from build123d import *

# Parameters (mm, degrees)
SKETCH1_R           = 10
SKETCH1_R_2         = 7.5
BOSS_EXTRUDE1_DEPTH = 25
THREAD1_PITCH       = 0.3175
SKETCH4_W           = 146
SKETCH4_H           = 146
BOSS_EXTRUDE2_DEPTH = 2
SKETCH5_W           = 148
SKETCH5_H           = 148
BOSS_EXTRUDE3_DEPTH = 1
SKETCH6_W           = 10
SKETCH6_H           = 3
SKETCH6_R           = 1
BOSS_EXTRUDE4_DEPTH = 5
CHAMFER2_START      = -5
CHAMFER2_DEPTH      = 10
SKETCH9_R           = 10
CUT_EXTRUDE1_DEPTH  = 111.385687501
FILLET1_R           = 1


with BuildPart() as part:
    # Sketch1 → Boss-Extrude1 (new body)
    with BuildSketch(Plane(origin=(0, 0, 0), x_dir=(1, 0, 0), z_dir=(0, 1, 0))):
        with Locations(Location((0, 0, 0), (0, 0, 270))):
            Circle(SKETCH1_R)
        with Locations(Location((0, 0, 0), (0, 0, 270))):
            Circle(SKETCH1_R_2, mode=Mode.SUBTRACT)
    extrude(amount=BOSS_EXTRUDE1_DEPTH)

    # Thread1: arcs per turn and ends read off the stored shape
    # Thread1: the profile of Thread Profile1 profile screwed along a right-hand helix through 18.897638 turns, 6 arcs to a turn; built about Z, then put on its axis
    thread1_z = Axis((0, 0, 0), (0, 0, 1))
    thread1_corners = [(10.0003, 0, -0.000173205), (10.0003, 0, 0.277985704), (9.828148085, 0, 0.17859375), (9.828148085, 0, 0.09921875)]
    with BuildLine(mode=Mode.PRIVATE) as thread1_profile:
        Line(thread1_corners[0], thread1_corners[1])
        Line(thread1_corners[1], thread1_corners[2])
        Line(thread1_corners[2], thread1_corners[3])
        Line(thread1_corners[3], thread1_corners[0])
    thread1_cap = Face(thread1_profile.wire())
    thread1_turn_angles = [0, 30, 60, 90, 120, 150, 180, 210, 240, 270, 300, 330, 360]
    thread1_turn_weights = [1, 0.8660254037844387, 1, 0.8660254037844387, 1, 0.8660254037844387, 1, 0.8660254037844387, 1, 0.8660254037844387, 1, 0.8660254037844387, 1]
    thread1_turn_rails = [Edge.make_bspline([Vector(p[0], p[1], 0).rotate(thread1_z, thread1_turn_angles[k]) / thread1_turn_weights[k] + Vector(0, 0, p[2] + THREAD1_PITCH * thread1_turn_angles[k] / 360) for k in range(13)], [0, 0, 0, 1, 1, 2, 2, 3, 3, 4, 4, 5, 5, 6, 6, 6], 2, thread1_turn_weights) for p in thread1_corners]
    thread1_turn_sides = [Face.make_surface_from_curves(thread1_turn_rails[p[0]], thread1_turn_rails[p[1]]) for p in [(0, 1), (1, 2), (2, 3), (3, 0)]]
    thread1_last_angles = [6480, 6510, 6540, 6570, 6600, 6630, 6660, 6690, 6720, 6750, 6780, 6791.57480315, 6803.149606299]
    thread1_last_weights = [1, 0.8660254037844387, 1, 0.8660254037844387, 1, 0.8660254037844387, 1, 0.8660254037844387, 1, 0.8660254037844387, 1, 0.9796635825089068, 1]
    thread1_last_rails = [Edge.make_bspline([Vector(p[0], p[1], 0).rotate(thread1_z, thread1_last_angles[k]) / thread1_last_weights[k] + Vector(0, 0, p[2] + THREAD1_PITCH * thread1_last_angles[k] / 360) for k in range(13)], [0, 0, 0, 1, 1, 2, 2, 3, 3, 4, 4, 5, 5, 6, 6, 6], 2, thread1_last_weights) for p in thread1_corners]
    thread1_last_sides = [Face.make_surface_from_curves(thread1_last_rails[p[0]], thread1_last_rails[p[1]]) for p in [(0, 1), (1, 2), (2, 3), (3, 0)]]
    thread1 = Plane(origin=(0, -0.5, 0), x_dir=(1, 0, 0), z_dir=(0, 1, 0)) * Solid(Shell([*[p.moved(Location((0, 0, THREAD1_PITCH * i))) for i in range(18) for p in thread1_turn_sides], *thread1_last_sides, thread1_cap, thread1_cap.rotate(thread1_z, 6803.149606299).moved(Location((0, 0, THREAD1_PITCH * 6803.149606299 / 360)))]))
    add(thread1, mode=Mode.SUBTRACT)

    # Sketch4 → Boss-Extrude2 (add)
    with BuildSketch(Plane(origin=(0, 25, 0), x_dir=(1, 0, 0), z_dir=(0, 1, 0))):
        Rectangle(SKETCH4_W, SKETCH4_H)
    extrude(amount=BOSS_EXTRUDE2_DEPTH)

    # Sketch5 → Boss-Extrude3 (add)
    with BuildSketch(Plane.XZ.offset(-25)):
        Rectangle(SKETCH5_W, SKETCH5_H)
    extrude(amount=-BOSS_EXTRUDE3_DEPTH)

    # Sketch6 → Boss-Extrude4 (add, symmetric)
    with BuildSketch(Plane.XY):
        with Locations((73, 23.5)):
            Rectangle(SKETCH6_W, SKETCH6_H)
        with Locations((76, 23.5)):
            Circle(SKETCH6_R, mode=Mode.SUBTRACT)
    extrude(amount=BOSS_EXTRUDE4_DEPTH, both=True)

    # Chamfer2: read off the stored shape, not the designer's step
    # Chamfer2 outline → Chamfer2 (add)
    with BuildSketch(Plane.XY.offset(CHAMFER2_START)):
        Polygon((68, 25), (65, 25), (68, 22), align=None)
    extrude(amount=CHAMFER2_DEPTH)

    # Sketch9 → Cut-Extrude1 (cut, through all)
    with BuildSketch(Plane.XZ.offset(-25)):
        Circle(SKETCH9_R)
    extrude(amount=CUT_EXTRUDE1_DEPTH, mode=Mode.SUBTRACT)

    # Fillet1
    fillet1_edges = [part.edges().sort_by_distance(p)[0] for p in [
        (78, 22, 0),
        (78, 25, 0),
    ]]
    fillet(fillet1_edges, radius=FILLET1_R)


solid = part.part
Part model, mm, in its own coordinate system. Give positions to 0.01 mm unless a question says otherwise; leave off trailing zeros. Loops run counter-clockwise (first coordinate to the right, second up) from the corner with the lowest first, then second, coordinate; pieces in that order, holes last. Notation, with made-up numbers: M 26,88 L 61,88 A34 cw 61,121 Z; hole C -6.5,86 d2. An arc over 180 degrees is marked long. Put each result on its own line as item: value. Start each with the question number.
1) Probe probe 1 along Y at (x, z) = (76, 1); probe 2 along Y at (x, z) = (-66, -21); probe 3 along Z at (x, y) = (-19.5, 26.35). List the from-to ranges inside material, lowest first.
2) Flat gauge pins, fed straight in: pin 1 (1.1 mm diameter, centred on y = 26.5, z = 1.5, fed in from -X); pin 2 (2 mm diameter, centred on y = 26.5, z = -41, fed in from +X); pin 3 (0.5 mm diameter, centred on y = 26.5, z = 19, fed in from +X); pin 4 (10 mm diameter, centred on x = 36, z = -16.5, fed in from -Y). Where does each tip first touch, or does it go through?
3) Saw through at A-A (z = -39). List the corners of the cut face in (x, y).
4) Saw through at B-B (x = 33). List the corners of the cut face in (y, z).
5) Saw through at C-C (z = -3). List the corners of the cut face in (x, y), then the cut area to 3 significant figures.
Numbers:
1. probe 1: 22 to 22.5, 24.5 to 25
1. probe 2: 25 to 27
1. probe 3: -73 to 73
2. pin 1: x = -74
2. pin 2: x = 74
2. pin 3: x = 73
2. pin 4: y = 25
3. outline: M -74,25 L 74,25 L 74,26 L 73,26 L 73,27 L -73,27 L -73,26 L -74,26 Z
4. outline: M 25,-74 L 26,-74 L 26,-73 L 27,-73 L 27,73 L 26,73 L 26,74 L 25,74 Z
5. outline: M -74,25 L 65,25 L 68,22 L 77,22 A1 ccw 78,23 L 78,24 A1 ccw 77,25 L 74,25 L 74,26 L 73,26 L 73,27 L -73,27 L -73,26 L -74,26 Z; hole C 76,23.5 d2
5. area: 325 mm^2
